Read the model definition and answer for the solid it produces. Units are mm, in the model's axes. Round coordinates to 2 decimals unless told otherwise and drop trailing zeros. Loops run counter-clockwise (first coordinate to the right, second up) from the corner with the lowest first, then second, coordinate; pieces in that order, holes last. Notation, with made-up numbers: (73, 57) - (104, 57) arc R10 cw to (104, 64) - close; hole circle Ø5 at (76, 83). An arc over 180 degrees is marked (long way). Use one line per item in the form item = value. Start each with the question number.
```python
from build123d import *

# Parameters (mm, degrees)
F1_DEPTH = 63.246
F2_R     = 5.08
F3_W     = 42.474462
F3_H     = 53.623985
F4_DEPTH = 1.27


with BuildPart() as f1:
    # F0 (on Front) → F1 (new body)
    with BuildSketch(Plane.XZ):
        Polygon((-46.401739, 1.929175), (-46.401739, 0), (48.229381, 0), (48.229381, 6.193668), align=None)
    extrude(amount=F1_DEPTH)

    # F2
    f2_edges = [f1.edges().sort_by_distance(p)[0] for p in [
        (48.229381, 0, 3.096834),
        (48.229381, -63.246, 3.096834),
        (-46.401739, -63.246, 0.964588),
        (-46.401739, 0, 0.964588),
    ]]
    fillet(f2_edges, radius=F2_R)

    # F3 (on face) → F4 (join)
    with BuildSketch(Plane(origin=(-0.180802, 0, 4.012093), x_dir=(0.998986, 0, 0.045019), z_dir=(-0.045019, 0, 0.998986))):
        with Locations((17.051772, -31.891992)):
            Rectangle(F3_W, F3_H)
    extrude(amount=-F4_DEPTH)


solid = f1.part
```
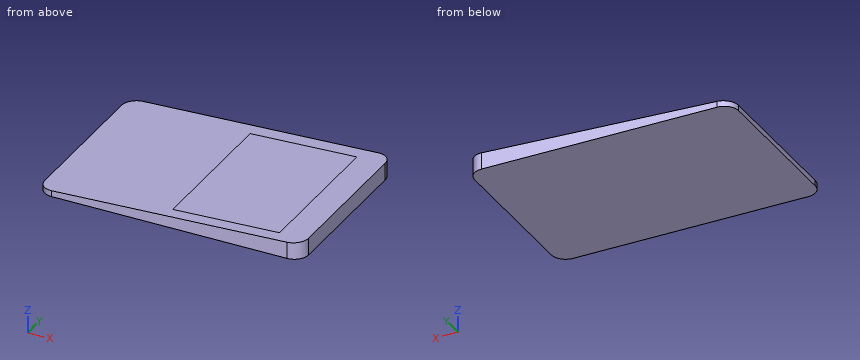
1) A flat-ended cylindrical pin translates along its axis: pin 1 (0.5 mm diameter, centred on x = 11.5, z = 5, fed in from +Y). Find the tip coordinate at first contact, or state that the pin passes through.
2) A cutting plane is placed at D-D on x = -1.5. Write down the section's boundary in (y, z).
3) Straight lines are drawn through the part: line 1 (Z direction, x = -2, y = -39); line 2 (Z direction, x = 14.5, y = -17); line 3 (X direction, y = -4, z = 1). For each, find the intervals that lie inside material, in ascending order. Write a range as from..to.
Checks:
q1.pin_1 = through
q2.outline = (-63.25, 0) - (0, 0) - (0, 3.95) - (-63.25, 3.95) - close
q3.line_1 = 0..3.93
q3.line_2 = 0..4.67
q3.line_3 = -46.29..48.11
